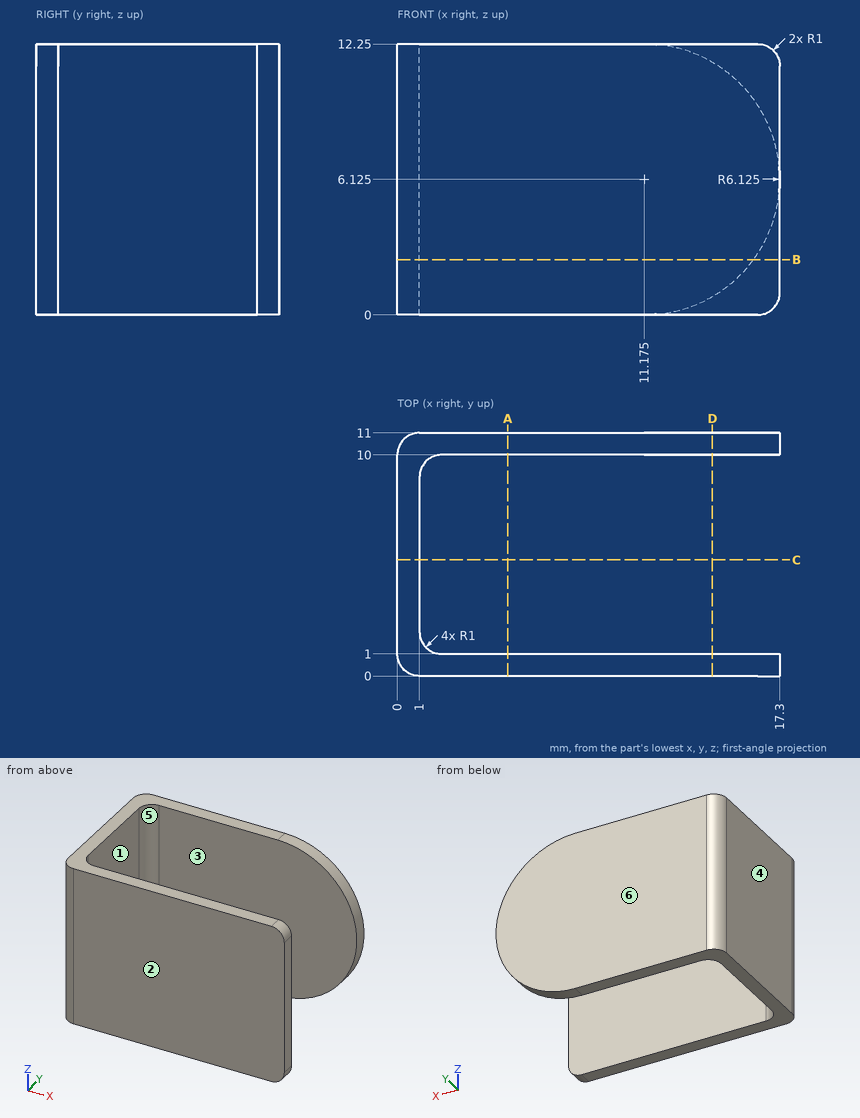
Drawing for the job (mm, zero at the part's lowest x, y, z). A direction names the side the tool comes from. Give positions to 0.01 mm unless a question says otherwise; leave off trailing zeros. Loops run counter-clockwise (first coordinate to the right, second up) from the corner with the lowest first, then second, coordinate; pieces in that order, holes last.
(1) Pin check, flat tips, straight feed: pin 1 (5.5 mm diameter, centred on y = 7, z = 6, fed in from +X); pin 2 (2 mm diameter, centred on y = 3, z = 8.5, fed in from +X). Stop position of each tip, or through.
Return value:
pin 1: stops at x = 1.34
pin 2: stops at x = 1
(2) Pull direction Y, two halves, no side cores. Call the marked faces 1, 2, 3 and 4: pulls with the +Y half, pulls with the -Y half, needs draft (parallel to the pull), parting line crosses it, or undercut.
Return value:
face 1: undercut
face 2: pulls with the -Y half
face 3: undercut
face 4: needs draft
(3) Drill centre lines: line 1 along Y through (x, z) = (10.5, 3); line 2 along X through (y, z) = (7.75, 2.75); line 3 along Z through (x, y) = (11.5, 10.25). Where is each one in solid material? Low to high.
Return value:
line 1: y = 0 to 1, 10 to 11
line 2: x = 0 to 1
line 3: z = 0.01 to 12.24
(4) Band-saw the part on C-C (y = 5.25). Write the cut outline in (x, z), and give its area (4 significant figures).
Return value:
outline: (0, 0) - (1, 0) - (1, 12.25) - (0, 12.25) - close
area: 12.25 mm2
(5) Band-saw the part on B-B (z = 2.5). Write the cut outline in (x, y).
Return value:
outline: (0, 1) arc R1 ccw to (1, 0) - (17.3, 0) - (17.3, 1) - (2, 1) arc R1 cw to (1, 2) - (1, 9) arc R1 cw to (2, 10) - (16.11, 10) - (16.11, 11) - (1, 11) arc R1 ccw to (0, 10) - close
(6) 3-axis set-ups, long thin cutter, end or side, ignore diameter. For the marked faces 5 and 6: which of +Z, -Z, +X, -X, +Y, -Y reach the whole face in a straight line?
Return value:
face 5: +Z, -Z, +X
face 6: +Z, -Z, +X, -X, +Y
(7) Band-saw the part on D-D (x = 14.25). Write the cut outline in (y, z), and give its area (3 significant figures).
Return value:
outline: (0, 0) - (1, 0) - (1, 12.25) - (0, 12.25) - close; (10, 0.83) - (11, 0.83) - (11, 11.42) - (10, 11.42) - close
area: 22.8 mm2
(8) Band-saw the part on A-A (x = 5). Write the cut outline in (y, z).
Return value:
outline: (0, 0) - (1, 0) - (1, 12.25) - (0, 12.25) - close; (10, 0) - (11, 0) - (11, 12.25) - (10, 12.25) - close
